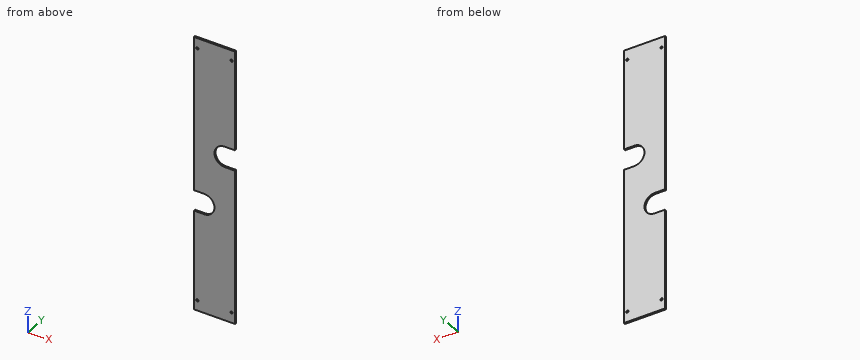
```python
from build123d import *

# Parameters (mm, degrees)
SKETCH1_W           = 76.2
SKETCH1_H           = 3.175
BOSS_EXTRUDE1_DEPTH = 508
CUT_EXTRUDE1_DEPTH  = 4.175
SKETCH4_R           = 2.0828
CUT_EXTRUDE2_DEPTH  = 4.175


with BuildPart() as part:
    # Sketch1 → Boss-Extrude1 (new body)
    with BuildSketch(Plane.XY):
        with Locations((0, 21.307750599)):
            Rectangle(SKETCH1_W, SKETCH1_H)
    extrude(amount=BOSS_EXTRUDE1_DEPTH)

    # Sketch2 → Cut-Extrude1 (cut, through all)
    with BuildSketch(Plane(origin=(0, 22.895250599, 0), x_dir=(1, 0, 0), z_dir=(0, 1, 0))):
        with BuildLine():
            Line((-19.05, -184.15), (-38.1, -184.15))
            Line((-38.1, -184.15), (-38.1, -222.25))
            Line((-38.1, -222.25), (-19.05, -222.25))
            ThreePointArc((-19.05, -222.25), (0, -203.2), (-19.05, -184.15))
        make_face()
        with BuildLine():
            Line((19.05, -323.85), (38.1, -323.85))
            Line((38.1, -323.85), (38.1, -285.75))
            Line((38.1, -285.75), (19.05, -285.75))
            ThreePointArc((19.05, -285.75), (0, -304.8), (19.05, -323.85))
        make_face()
    extrude(amount=-CUT_EXTRUDE1_DEPTH, mode=Mode.SUBTRACT)

    # Sketch4 → Cut-Extrude2 (cut, through all)
    with BuildSketch(Plane(origin=(0, 22.895250599, 0), x_dir=(1, 0, 0), z_dir=(0, 1, 0))):
        with Locations((-31.75, -488.95)):
            Circle(SKETCH4_R)
        with Locations((31.75, -19.05)):
            Circle(SKETCH4_R)
    cut_extrude2 = extrude(amount=-CUT_EXTRUDE2_DEPTH, mode=Mode.SUBTRACT)

    # Mirror2: Cut-Extrude2 across plane
    add(cut_extrude2.mirror(Plane.XY.offset(254)), mode=Mode.SUBTRACT)


solid = part.part
```
Geometry check sheet. Reference: the model listing, model coordinates, mm. Round coordinates to 2 decimals unless told otherwise and drop trailing zeros. Loops run counter-clockwise (first coordinate to the right, second up) from the corner with the lowest first, then second, coordinate; pieces in that order, holes last. Notation, with made-up numbers: (-12.75, 53.5) - (8.25, 53.5) arc R11 ccw to (8.25, 65.5) - close; hole circle Ø3 at (-26, 11.25). An arc over 180 degrees is marked (long way). Use a Markdown table: item, result.
Q1. Cross-section at C-C on z = 203.2. Record the cut outline in (x, y), plus the area to 3 significant figures.
Solutions:
| item | result |
|---|---|
| outline | (0, 19.72) - (38.1, 19.72) - (38.1, 22.9) - (0, 22.9) - close |
| area | 121 mm2 |
Q2. Material ranges on line 1 (X direction, y = 21.95, z = 488.95); line 2 (Z direction, x = 31.75, y = 21.8); line 3 (Z direction, x = -31.75, y = 21.65), recorded low to high.
Solutions:
| item | result |
|---|---|
| line 1 | x = -38.1 to -33.83, -29.67 to 29.67, 33.83 to 38.1 |
| line 2 | z = 0 to 16.97, 21.13 to 285.75, 323.85 to 486.87, 491.03 to 508 |
| line 3 | z = 0 to 16.97, 21.13 to 184.15, 222.25 to 486.87, 491.03 to 508 |
Q3. Cross-section at B-B on x = -5.5. Record the cut outline in (y, z), plus the area to 3 significant figures.
Solutions:
| item | result |
|---|---|
| outline | (19.72, 0) - (22.9, 0) - (22.9, 189.81) - (19.72, 189.81) - close; (19.72, 216.59) - (22.9, 216.59) - (22.9, 508) - (19.72, 508) - close |
| area | 1,530 mm2 |
Q4. Cross-section at D-D on z = 302. Record the cut outline in (x, y).
Solutions:
| item | result |
|---|---|
| outline | (-38.1, 19.72) - (0.21, 19.72) - (0.21, 22.9) - (-38.1, 22.9) - close |
Q5. Cross-section at A-A on y = 21.9. Record the cut outline in (x, z).
Solutions:
| item | result |
|---|---|
| outline | (-38.1, 0) - (38.1, 0) - (38.1, 285.75) - (19.05, 285.75) arc R19.05 cw to (19.05, 323.85) - (38.1, 323.85) - (38.1, 508) - (-38.1, 508) - (-38.1, 222.25) - (-19.05, 222.25) arc R19.05 cw to (-19.05, 184.15) - (-38.1, 184.15) - close; hole circle Ø4.17 at (-31.75, 19.05); hole circle Ø4.17 at (-31.75, 488.95); hole circle Ø4.17 at (31.75, 19.05); hole circle Ø4.17 at (31.75, 488.95) |
Q6. Go/stop test with a flat-tipped pin: P1, Ø3.5, axis at x = 31.75, z = 488.95, coming from the +Y side. Record where the tip stops, or that it passes through.
Solutions:
| item | result |
|---|---|
| P1 | passes through |
